The drawing under review shows one solid part. Ordinate dimensions are in mm from its lowest x, y, z. A direction names the side the tool comes from. Give positions to 0.01 mm unless a question says otherwise; leave off trailing zeros. Write each loop counter-clockwise with the first axis right and the second up, starting at its lowest first coordinate (ties: lowest second). Pieces come first, ordered by that corner, then holes.
Q1. Machinability: for the marked faces 1 and 2, which of the approach directions +Z, -Z, +X, -X, +Y, -Y give a long, thin tool a straight path to every point of the face, cutting with its end or side? Answer none if there is none.
Q2. Mouldability with a two-part tool opening along X and no side actions: class the marked faces 3, 4 and 5 as released by +X, released by -X, zero draft, split by the parting line, or undercut.
Q3. We need section D-D (z = 9.85). Write out the cut boundary in (x, y).
Q4. Insertion check: P1, Ø1.2, axis at x = 3, z = 25, coming from the +Y side; P2, Ø1, axis at x = 18.5, z = 27.5, coming from the -Y side. Each pin has a flat end and moves straight along its axis. Give the tip position at first contact, or say it passes through.
Q5. For line 1 (X direction, y = 8.65, z = 9.85); line 2 (Z direction, x = 3.5, y = 7.3); line 3 (X direction, y = 4.5, z = 21.5), list the stretches that pass through material, from the lowest coordinate up.
Q6. We need section B-B (z = 28). Write out the cut boundary in (x, y).
Q7. We need section C-C (x = 23.5). Write out the cut boundary in (y, z).
Q8. We need section A-A (y = 2.5). Write out the cut boundary in (x, z).
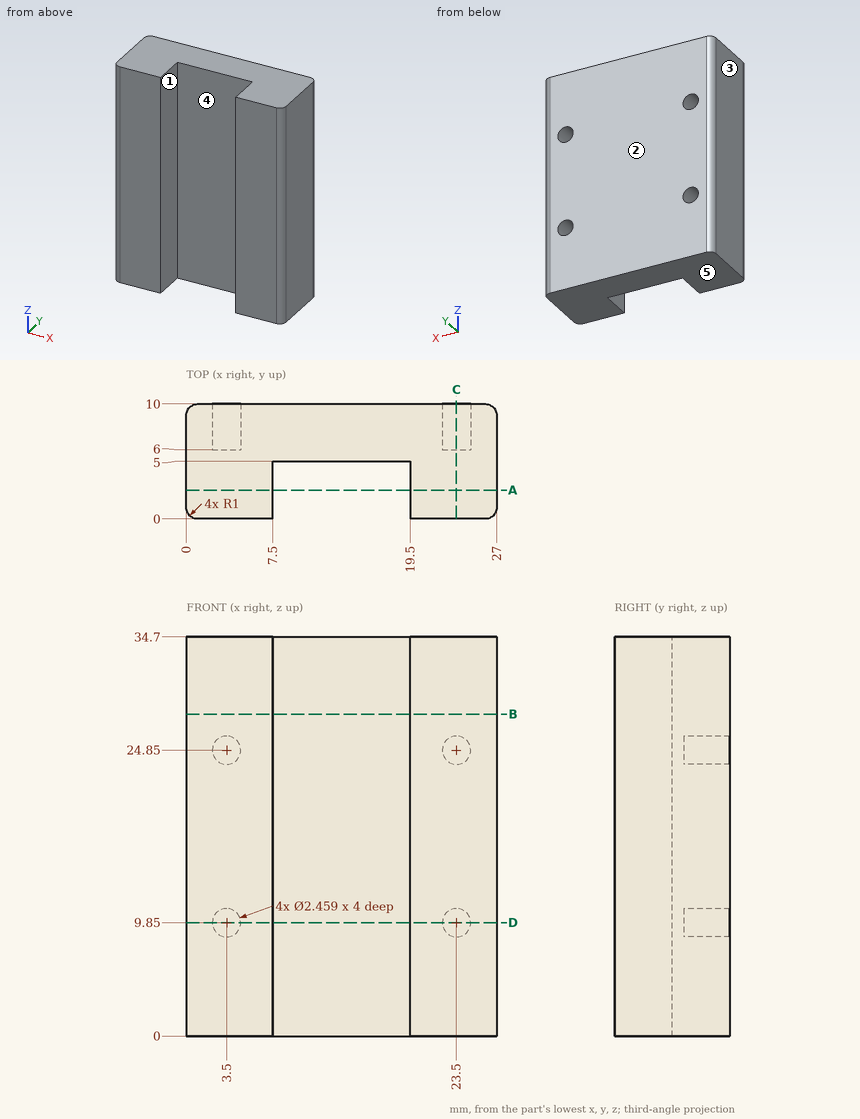
Computed:
1. face 1: +Z, -Z, -Y
1. face 2: +Z, -Z, +X, -X, +Y
2. face 3: released by -X
2. face 4: undercut
2. face 5: zero draft
3. outline: (0, 1) arc R1 ccw to (1, 0) - (7.5, 0) - (7.5, 5) - (19.5, 5) - (19.5, 0) - (26, 0) arc R1 ccw to (27, 1) - (27, 9) arc R1 ccw to (26, 10) - (24.73, 10) - (24.73, 6) - (22.27, 6) - (22.27, 10) - (4.73, 10) - (4.73, 6) - (2.27, 6) - (2.27, 10) - (1, 10) arc R1 ccw to (0, 9) - close
4. P1: stops at y = 6
4. P2: stops at y = 5
5. line 1: x = 0 to 2.27, 4.73 to 22.27, 24.73 to 27
5. line 2: z = 0 to 8.62, 11.08 to 23.62, 26.08 to 34.7
5. line 3: x = 0 to 7.5, 19.5 to 27
6. outline: (0, 1) arc R1 ccw to (1, 0) - (7.5, 0) - (7.5, 5) - (19.5, 5) - (19.5, 0) - (26, 0) arc R1 ccw to (27, 1) - (27, 9) arc R1 ccw to (26, 10) - (1, 10) arc R1 ccw to (0, 9) - close
7. outline: (0, 0) - (10, 0) - (10, 8.62) - (6, 8.62) - (6, 11.08) - (10, 11.08) - (10, 23.62) - (6, 23.62) - (6, 26.08) - (10, 26.08) - (10, 34.7) - (0, 34.7) - close
8. outline: (0, 0) - (7.5, 0) - (7.5, 34.7) - (0, 34.7) - close; (19.5, 0) - (27, 0) - (27, 34.7) - (19.5, 34.7) - close
